Can you work these out from the model? Positions are in its coordinate system, mm. Face numbers are marked on the shaded views. Round coordinates to 2 decimals unless told otherwise and drop trailing zeros. Order: outer loops, then holes, each group sorted by start corner. A loop starts at its lowest first (then second) coordinate and runs counter-clockwise, first axis right, second up. Notation, with made-up numbers: (-17.75, 78.5) - (9.25, 78.5) arc R22 cw to (9.25, 84.5) - close; hole circle Ø7 at (80, -18.5). An arc over 180 degrees is marked (long way). Write item = value, one per line.
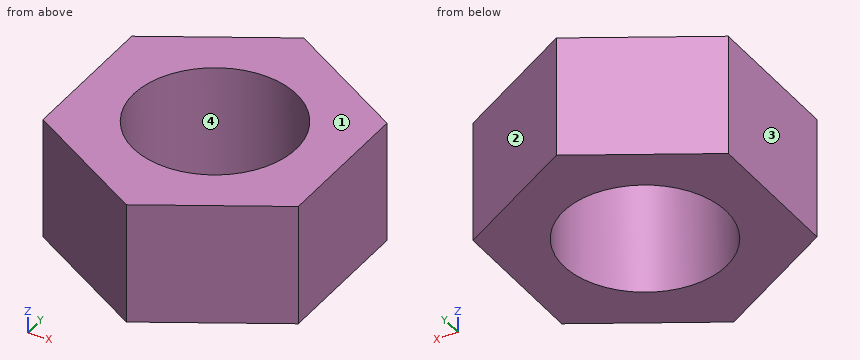
from build123d import *

# Parameters (mm, degrees)
EXTRUDE_1_DEPTH     = 10.5
SKETCH_2_R          = 7
CUT_EXTRUDE_1_DEPTH = 10.5


with BuildPart() as part:
    # 草图1 → 凸台-拉伸1 (new body)
    with BuildSketch(Plane.XY):
        Polygon((37.315481106, 15.159530396), (37.315481106, 2.457824474), (26.315481106, -3.893028487), (15.315481106, 2.457824474), (15.315481106, 15.159530396), (26.315481106, 21.510383357), align=None)
    extrude(amount=EXTRUDE_1_DEPTH)

    # 草图2 → 切除-拉伸1 (cut)
    with BuildSketch(Plane(origin=(0, 0, 0), x_dir=(-1, 0, 0), z_dir=(0, 0, -1))):
        with Locations((-26.315481106, 8.808677435)):
            Circle(SKETCH_2_R)
    extrude(amount=-CUT_EXTRUDE_1_DEPTH, mode=Mode.SUBTRACT)


solid = part.part
(1) Will these pins go through, and if not, where does the flat tip stop? P1, Ø3, axis at y = 1.5, z = 5, coming from the -X side; P2, Ø11, axis at x = 26.32, y = 8.81, coming from the -Z side; P3, Ø4, axis at x = 21, z = 3.5, coming from the -Y side.
Computed:
P1 = 15.32
P2 = through
P3 = -1.98
(2) If we section it at A-A (y = 4.5): Write out the boundary of the cut face in (x, z).
Computed:
outline = (15.32, 0) - (20.8, 0) - (20.8, 10.5) - (15.32, 10.5) - close; (31.83, 0) - (37.32, 0) - (37.32, 10.5) - (31.83, 10.5) - close
(3) If we section it at C-C (z = 4.25): Write out the boundary of the cut face in (x, y).
Computed:
outline = (15.32, 2.46) - (26.32, -3.89) - (37.32, 2.46) - (37.32, 15.16) - (26.32, 21.51) - (15.32, 15.16) - close; hole circle Ø14 at (26.32, 8.81)
(4) Thinking about a two-plate mould opening in X: for the marked faces 1, 2, 3 and 4, which applies, +X half, -X half, draft (parallel to the pull), parting line (faces both ways), or undercut?
Computed:
face_1 = draft
face_2 = +X half
face_3 = -X half
face_4 = undercut
(5) If I drill on line 1 (Y direction, x = 20, z = 6.5); line 2 (X direction, y = 14.5, z = 1); line 3 (X direction, y = 13, z = 9.75), over which ranges is the centre line in solid material (lowest first)? Write a range as from..to.
Computed:
line_1 = -0.25..5.79, 11.83..17.86
line_2 = 15.32..22.24, 30.39..37.32
line_3 = 15.32..20.71, 31.92..37.32
(6) If we section it at D-D (y = -1.75): Write out the boundary of the cut face in (x, z), plus the area to 3 significant figures.
Computed:
outline = (22.6, 0) - (30.03, 0) - (30.03, 10.5) - (22.6, 10.5) - close
area = 77.9 mm^2
(7) If we section it at B-B (x = 20.5): Write out the boundary of the cut face in (y, z), plus the area to 3 significant figures.
Computed:
outline = (-0.54, 0) - (4.91, 0) - (4.91, 10.5) - (-0.54, 10.5) - close; (12.7, 0) - (18.15, 0) - (18.15, 10.5) - (12.7, 10.5) - close
area = 114 mm^2
